from build123d import *

# Parameters (mm, degrees)
CYLINDER008_R     = 3
CYLINDER008_DEPTH = 1.1
CYLINDER007_R     = 3
CYLINDER007_DEPTH = 1.1
CYLINDER004_R     = 2.4
CYLINDER004_DEPTH = 13
CYLINDER005_R     = 2.7
CYLINDER005_DEPTH = 1
CYLINDER006_R     = 2.7
CYLINDER006_DEPTH = 1
CYLINDER003_R     = 2.4
CYLINDER003_DEPTH = 13
CYLINDER002_R     = 0.7
CYLINDER002_DEPTH = 16
BOX007_W          = 12.25
BOX007_H          = 10
BOX007_DEPTH      = 10
BOX003_W          = 12.25
BOX003_H          = 23.78
BOX003_DEPTH      = 22.68
BOX008_W          = 24.3
BOX008_H          = 21
BOX008_DEPTH      = 30


with BuildPart() as cylinder008:
    # Cylinder008 → Cylinder008 (new body)
    with BuildSketch(Plane(origin=(-2.5, 17.5, -0.1), x_dir=(1, 0, 0), z_dir=(0, 0, 1))):
        Circle(CYLINDER008_R)
    extrude(amount=CYLINDER008_DEPTH)


with BuildPart() as fusion005:
    # Cylinder007 → Cylinder007 (new body)
    with BuildSketch(Plane(origin=(14.74, 17.5, -0.1), x_dir=(1, 0, 0), z_dir=(0, 0, 1))):
        Circle(CYLINDER007_R)
    extrude(amount=CYLINDER007_DEPTH)

    # Fusion005: union Cylinder008
    add(cylinder008.part)


with BuildPart() as cylinder004:
    # Cylinder004 → Cylinder004 (new body)
    with BuildSketch(Plane(origin=(14.74, 17.5, -6.5), x_dir=(1, 0, 0), z_dir=(0, 0, 1))):
        Circle(CYLINDER004_R)
    extrude(amount=CYLINDER004_DEPTH)


with BuildPart() as cylinder005:
    # Cylinder005 → Cylinder005 (new body)
    with BuildSketch(Plane(origin=(-2.5, 17.5, 6.5), x_dir=(1, 0, 0), z_dir=(0, 0, 1))):
        Circle(CYLINDER005_R)
    extrude(amount=CYLINDER005_DEPTH)


with BuildPart() as cylinder006:
    # Cylinder006 → Cylinder006 (new body)
    with BuildSketch(Plane(origin=(14.74, 17.5, 6.5), x_dir=(1, 0, 0), z_dir=(0, 0, 1))):
        Circle(CYLINDER006_R)
    extrude(amount=CYLINDER006_DEPTH)


with BuildPart() as fusion006:
    # Cylinder003 → Cylinder003 (new body)
    with BuildSketch(Plane(origin=(-2.5, 17.5, -6.5), x_dir=(1, 0, 0), z_dir=(0, 0, 1))):
        Circle(CYLINDER003_R)
    extrude(amount=CYLINDER003_DEPTH)

    # Fusion004: union Cylinder004, Cylinder005, Cylinder006
    add(cylinder004.part)
    add(cylinder005.part)
    add(cylinder006.part)


with BuildPart() as fusion006_1:
    # Fusion004 placement: moved
    add(fusion006.part.moved(Location((0, 0, 1))))

    # Fusion006: union Fusion005
    add(fusion005.part)


with BuildPart() as cylinder002:
    # Cylinder002 → Cylinder002 (new body)
    with BuildSketch(Plane(origin=(6, 22, 25), x_dir=(1, 0, 0), z_dir=(0, -1, 0))):
        Circle(CYLINDER002_R)
    extrude(amount=CYLINDER002_DEPTH)


with BuildPart() as cube004:
    # Box007 → Box007 (new body)
    with BuildSketch(Plane(origin=(0, -3.25, 22), x_dir=(1, 0, 0), z_dir=(0, 0, 1))):
        with Locations((6.125, 5)):
            Rectangle(BOX007_W, BOX007_H)
    extrude(amount=BOX007_DEPTH)


with BuildPart() as servo002:
    # Box003 → Box003 (new body)
    with BuildSketch(Plane(origin=(0, -1, 0), x_dir=(1, 0, 0), z_dir=(0, 0, 1))):
        with Locations((6.125, 11.89)):
            Rectangle(BOX003_W, BOX003_H)
    extrude(amount=BOX003_DEPTH)

    # Fusion002: union Cube004
    add(cube004.part)


with BuildPart() as fusion003:
    # Fusion003 base: copy of Cube004
    add(cube004.part)

    # Fusion003: union servo002
    add(servo002.part)


with BuildPart() as cut005:
    # Box008 → Box008 (new body)
    with BuildSketch(Plane(origin=(-6, 0, 0), x_dir=(1, 0, 0), z_dir=(0, 0, 1))):
        with Locations((12.15, 10.5)):
            Rectangle(BOX008_W, BOX008_H)
    extrude(amount=BOX008_DEPTH)

    # Cut002: cut Fusion003
    add(fusion003.part, mode=Mode.SUBTRACT)

    # Cut003: cut Cylinder002
    add(cylinder002.part, mode=Mode.SUBTRACT)

    # Cut005: cut Fusion006
    add(fusion006_1.part, mode=Mode.SUBTRACT)


with BuildPart() as cut005_1:
    # Cut005 placement: moved
    add(cut005.part.moved(Location((10, -17.5, 2))))


solid = cut005_1.part
Could you check a few things on this model? Use its own coordinates, in mm. A direction names the side the tool comes from. Give positions to 0.01 mm unless a question says otherwise; leave off trailing zeros. Write each loop counter-clockwise with the first axis right and the second up, starting at its lowest first coordinate (ties: lowest second). Pieces come first, ordered by that corner, then holes. Notation, with made-up numbers: (0, 13) -> (25, 13) arc R12 cw to (25, 31) -> close; hole circle Ø1 at (35, -26.5). An arc over 180 degrees is marked (long way). Write each question's results on one line, items separated by ' | '. Start each with the question number.
Q1. I'm going to push flat-ended pins straight in: pin 1 Ø2 at (x, z) = (16.5, 26.5) entering from -Y; pin 2 Ø3 at (x, y) = (24.74, 0) entering from -Z; pin 3 Ø6 at (x, y) = (16, -12.5) entering from -Z; pin 4 Ø1.1 at (x, z) = (16, 27) entering from -Y. Where does each tip first touch, or does it pass through?
Q2. Suppose I cut it at D-D, the plane y = -14. List the corners of the cut face in (x, z) for me, and give its area (4 significant figures).
Q3. Which directions (+Z, -Z, +X, -X, +Y, -Y) give clear straight access to the entire face, cutting with the end or side of a thin tool? Please do faces 1 (the face through (26.81, -1.54, 3)), 2 (the face through (19, 3.5, 27)), 3 (the face through (25, 0, 10.5)).
Q4. Suppose I cut it at C-C, the plane z = 6. List the corners of the cut face in (x, y) for me, and give its area (3 significant figures).
Q5. I need wall thicknesses on probe 1 along Y at (x, z) = (24.74, 2.4); probe 2 along X at (y, z) = (2.5, 5); probe 3 along Y at (x, z) = (24.74, 4.75). Which ranges of each line are inside material? Lowest first, please.
Q6. Suppose I cut it at B-B, the plane y = 0. State how many separate pieces and enclosed holes the cut face has, and give its area (3 significant figures).
Q7. Suppose I cut it at A-A, the plane z = 23.5. List the corners of the cut face in (x, y) for me.
Q8. We'd pull the mould along X, two halves only. Please class faces 4 (the face through (4, -7, 17)), 5 (the face through (16, -10.75, 28)), 6 (the face through (28.3, -7, 17)), 7 (the face through (16, -5, 32)): +X half, -X half, draft (parallel to the pull), parting line (faces both ways), or undercut.
Outcome:
1) pin 1: y = -10.75 | pin 2: z = 10.5 | pin 3: z = 24.68 | pin 4: through
2) outline: (4, 2) -> (10, 2) -> (10, 32) -> (4, 32) -> close; (22.25, 2) -> (28.3, 2) -> (28.3, 32) -> (22.25, 32) -> close | area: 361.5 mm2
3) face 1: -Z | face 2: +Z, -Z, +X, -X, +Y | face 3: none
4) outline: (4, -17.5) -> (10, -17.5) -> (10, 3.5) -> (4, 3.5) -> close; (22.25, -17.5) -> (28.3, -17.5) -> (28.3, 3.5) -> (22.25, 3.5) -> close; hole circle Ø4.8 at (7.5, 0); hole circle Ø4.8 at (24.74, 0) | area: 217 mm2
5) probe 1: -17.5 to -3, 3 to 3.5 | probe 2: 4 to 10, 22.25 to 28.3 | probe 3: -17.5 to -2.4, 2.4 to 3.5
6) separate pieces: 3 | enclosed holes: 1 | area: 366 mm2
7) outline: (4, -17.5) -> (10, -17.5) -> (10, 3.5) -> (4, 3.5) -> close; (22.25, -17.5) -> (28.3, -17.5) -> (28.3, 3.5) -> (22.25, 3.5) -> close
8) face 4: -X half | face 5: undercut | face 6: +X half | face 7: draft
